Can you work these out from the model? Positions are in its coordinate system, mm. A direction names the side the tool comes from. Give positions to 0.01 mm unless a question says otherwise; leave off trailing zeros. Write each loop counter-clockwise with the first axis right and the second up, starting at its lowest first coordinate (ties: lowest second). Pieces come first, ordered by that corner, then holes. Notation, with made-up numbers: (-29, 15) -> (-16, 15) arc R27 ccw to (-16, 37) -> close; hole circle Ø5 at (42, 23.25). An arc over 180 degrees is marked (long way). One line per item, written item: value.
from build123d import *

# Parameters (mm, degrees)
SKETCH_1_W          = 200
SKETCH_1_H          = 460
EXTRUDE_1_DEPTH     = 8
SKETCH_2_R          = 30
CUT_EXTRUDE_1_DEPTH = 10
SKETCH_3_R          = 2.25
CUT_EXTRUDE_2_DEPTH = 10
SKETCH_4_R          = 4
CUT_EXTRUDE_3_DEPTH = 4.4


with BuildPart() as part:
    # 草图1 → 凸台-拉伸1 (new body)
    with BuildSketch(Plane.XY):
        with Locations((0, 230)):
            Rectangle(SKETCH_1_W, SKETCH_1_H)
    extrude(amount=EXTRUDE_1_DEPTH)

    # 草图2 → 切除-拉伸1 (cut)
    with BuildSketch(Plane(origin=(0, 0, 0), x_dir=(-1, 0, 0), z_dir=(0, 0, -1))):
        with Locations((0, 370)):
            Circle(SKETCH_2_R)
    extrude(amount=-CUT_EXTRUDE_1_DEPTH, mode=Mode.SUBTRACT)

    # 草图3 → 切除-拉伸2 (cut)
    with BuildSketch(Plane(origin=(0, 0, 0), x_dir=(-1, 0, 0), z_dir=(0, 0, -1))):
        with Locations((0, 411.5)):
            Circle(SKETCH_3_R)
        with Locations((29.344931419, 399.344931419)):
            Circle(SKETCH_3_R)
        with Locations((41.5, 370)):
            Circle(SKETCH_3_R)
        with Locations((29.344931419, 340.655068581)):
            Circle(SKETCH_3_R)
        with Locations((0, 328.5)):
            Circle(SKETCH_3_R)
        with Locations((-29.344931419, 340.655068581)):
            Circle(SKETCH_3_R)
        with Locations((-41.5, 370)):
            Circle(SKETCH_3_R)
        with Locations((-29.344931419, 399.344931419)):
            Circle(SKETCH_3_R)
    extrude(amount=-CUT_EXTRUDE_2_DEPTH, mode=Mode.SUBTRACT)

    # 草图4 → 切除-拉伸3 (cut)
    with BuildSketch(Plane.XY.offset(8)):
        with Locations((29.344931419, 399.344931419)):
            Circle(SKETCH_4_R)
        with Locations((41.5, 370)):
            Circle(SKETCH_4_R)
        with Locations((29.344931419, 340.655068581)):
            Circle(SKETCH_4_R)
        with Locations((0, 328.5)):
            Circle(SKETCH_4_R)
        with Locations((-29.344931419, 340.655068581)):
            Circle(SKETCH_4_R)
        with Locations((-41.5, 370)):
            Circle(SKETCH_4_R)
        with Locations((-29.344931419, 399.344931419)):
            Circle(SKETCH_4_R)
        with Locations((0, 411.5)):
            Circle(SKETCH_4_R)
    extrude(amount=-CUT_EXTRUDE_3_DEPTH, mode=Mode.SUBTRACT)


solid = part.part
1) For faces 1 (the face through (-1, 460, 4)), 2 (the face through (-29.87, 403.31, 5.83)), which set-ups out of +Z, -Z, +X, -X, +Y, -Y let a thin tool reach every point of the face, with its end or its side?
Answer list:
face 1: +Z, -Z, +X, -X, +Y
face 2: +Z
2) I need wall thicknesses on L1, parallel to X at y = 328.5, z = 5.95; L2, parallel to Y at x = 18, z = 3.5; L3, parallel to X at y = 394.5, z = 7.5. Which ranges of each line are inside material? Lowest first, please.
Answer list:
L1: x = -100 to -4, 4 to 100
L2: y = 0 to 346, 394 to 460
L3: x = -100 to -17.31, 17.31 to 100
3) If we section it at A-A (y = 387.5): Write out the boundary of the cut face in (x, z).
Answer list:
outline: (-100, 0) -> (-24.37, 0) -> (-24.37, 8) -> (-100, 8) -> close; (24.37, 0) -> (100, 0) -> (100, 8) -> (24.37, 8) -> close
4) If we section it at C-C (z = 5.5): State how many separate pieces and enclosed holes the cut face has, and give its area (3 significant figures).
Answer list:
separate pieces: 1
enclosed holes: 9
area: 88,800 mm^2
5) If we section it at B-B (x = -15): Write out the boundary of the cut face in (y, z).
Answer list:
outline: (0, 0) -> (344.02, 0) -> (344.02, 8) -> (0, 8) -> close; (395.98, 0) -> (460, 0) -> (460, 8) -> (395.98, 8) -> close
6) We'd pull the mould along X, two halves only. Please class faces 3 (the face through (43.346, 366.451, 5.831)), 4 (the face through (-100, 227, 4)), 5 (the face through (-1, 233, 8)): released by +X, released by -X, zero draft, split by the parting line, or undercut.
Answer list:
face 3: undercut
face 4: released by -X
face 5: zero draft
7) Will these pins go through, and if not, where does the flat tip stop? pin 1 (4 mm diameter, centred on x = -29.34, y = 340.66, fed in from -Z); pin 2 (5 mm diameter, centred on x = 41.5, y = 370, fed in from +Z).
Answer list:
pin 1: passes through
pin 2: stops at z = 3.6
